from build123d import *

# Parameters (mm, degrees)
SKETCH1_W               = 30
SKETCH1_H               = 30
MAIN_BODY_DEPTH         = 11
SKETCH2_W               = 17.84
SKETCH2_H               = 2.8
WIRE_HOLE_DEPTH         = 6
BOARD_CAVITY_DEPTH      = 3
BOARD_CAVITY_DEPTH_BACK = 17.2
SKETCH3_W               = 20.5
SKETCH3_H               = 3.6
SKETCH4_W               = 10
SKETCH4_H               = 10
LIGHT_BOX_DEPTH         = 2
SKETCH5_R               = 1.5
CUT_EXTRUDE4_DEPTH      = 20
SKETCH7_W               = 20.5
SKETCH7_H               = 3.6
CUT_EXTRUDE5_DEPTH      = 1
BOSS_EXTRUDE1_DEPTH     = 30
BOSS_EXTRUDE2_START     = 0.6
SKETCH11_W              = 10
SKETCH11_H              = 10
SKETCH11_R              = 1.5
BOSS_EXTRUDE2_DEPTH     = 0.6
SKETCH12_W              = 44.814636294
SKETCH12_H              = 7.577756332
CUT_EXTRUDE6_DEPTH      = 40


with BuildPart() as part:
    # Sketch1 → Main Body (new body)
    with BuildSketch(Plane(origin=(0, 0, 0), x_dir=(1, 0, 0), z_dir=(0, 1, 0))):
        Rectangle(SKETCH1_W, SKETCH1_H)
    extrude(amount=MAIN_BODY_DEPTH)

    # Sketch2 → Wire Hole (cut)
    with BuildSketch(Plane.XZ):
        with Locations((0, 8.6)):
            Rectangle(SKETCH2_W, SKETCH2_H)
    extrude(amount=-WIRE_HOLE_DEPTH, mode=Mode.SUBTRACT)

    # Sketch3 → Board Cavity (cut, two sides: drawn at the far end of the back side and taken through both)
    with BuildSketch(Plane.XY.offset(7.2).offset(-BOARD_CAVITY_DEPTH_BACK)):
        with Locations((0, 4.2)):
            Rectangle(SKETCH3_W, SKETCH3_H)
    extrude(amount=BOARD_CAVITY_DEPTH + BOARD_CAVITY_DEPTH_BACK, mode=Mode.SUBTRACT)

    # Sketch4 → Light Box (cut)
    with BuildSketch(Plane.XZ.offset(-6)):
        with Locations((0, 0.05)):
            Rectangle(SKETCH4_W, SKETCH4_H)
    extrude(amount=-LIGHT_BOX_DEPTH, mode=Mode.SUBTRACT)

    # Sketch5 → Cut-Extrude4 (cut)
    with BuildSketch(Plane.XZ.offset(-8)):
        with Locations(Location((0, 0, 0), (0, 0, 270))):
            Circle(SKETCH5_R)
    extrude(amount=-CUT_EXTRUDE4_DEPTH, mode=Mode.SUBTRACT)

    # Sketch7 → Cut-Extrude5 (cut)
    with BuildSketch(Plane.XY.offset(-10)):
        with Locations((0, 4.2)):
            Rectangle(SKETCH7_W, SKETCH7_H)
    extrude(amount=-CUT_EXTRUDE5_DEPTH, mode=Mode.SUBTRACT)

    # Sketch8 → Boss-Extrude1 (add)
    with BuildSketch(Plane(origin=(0, 0, -15), x_dir=(-1, 0, 0), z_dir=(0, 0, -1))):
        Polygon((-15, 5.5), (-15, 3.8), (-17.2, 3.8), (-17.2, 2.5), (-19.75, 2.5), (-19.75, 8.5), (-17.2, 8.5), (-17.2, 7.2), (-15, 7.2), align=None)
    boss_extrude1 = extrude(amount=-BOSS_EXTRUDE1_DEPTH)

    # Mirror1: Boss-Extrude1 across plane
    add(boss_extrude1.mirror(Plane(origin=(0, 0, 0), x_dir=(0, 0, 1), z_dir=(1, 0, 0))))

    # Sketch9 → Cut-Revolve6 (revolve, cut)
    with BuildSketch(Plane.XY, mode=Mode.PRIVATE) as cut_revolve6_sk:
        with BuildLine():
            Line((0, 67.971820098), (0, 8))
            Line((0, 8), (-1.3, 8))
            ThreePointArc((-1.3, 8), (-29.992954197, 38.621972793), (0, 67.971820098))
        make_face()
    revolve(cut_revolve6_sk.sketch.rotate(Axis((0, 0, 0), (0, -1, 0)), 90), axis=Axis((0, 0, 0), (0, -1, 0)), mode=Mode.SUBTRACT)

    # Sketch11 → Boss-Extrude2 (add)
    with BuildSketch(Plane.XZ.offset(-8).offset(BOSS_EXTRUDE2_START)):
        with Locations((0, 0.05)):
            Rectangle(SKETCH11_W, SKETCH11_H)
        with Locations(Location((0, 0, 0), (0, 0, 270))):
            Circle(SKETCH11_R, mode=Mode.SUBTRACT)
    extrude(amount=-BOSS_EXTRUDE2_DEPTH)

    # Sketch12 → Cut-Extrude6 (cut)
    with BuildSketch(Plane(origin=(0, 0, -15), x_dir=(-1, 0, 0), z_dir=(0, 0, -1))):
        with Locations((-2.128069321, 9.788878166)):
            Rectangle(SKETCH12_W, SKETCH12_H)
    extrude(amount=-CUT_EXTRUDE6_DEPTH, mode=Mode.SUBTRACT)


solid = part.part
Could you check a few things on this model? Use its own coordinates, in mm. A direction names the side the tool comes from. Round coordinates to 2 decimals unless told otherwise and drop trailing zeros. Write each loop counter-clockwise with the first axis right and the second up, starting at its lowest first coordinate (ties: lowest second). Pieces come first, ordered by that corner, then holes. Notation, with made-up numbers: (15, -1) - (29, -1) arc R28 ccw to (29, 19) - close; hole circle Ø8 at (-24.5, 39). An arc over 180 degrees is marked (long way). Use a Markdown table: item, result.
Q1. Please list where these lines run through material, in increasing order: L1, parallel to X at y = 5.15, z = 9.25; L2, parallel to Z at x = 6, y = 3.9; L3, parallel to X at y = 3.5, z = -11.75.
Output values:
| item | result |
|---|---|
| L1 | -19.75 to -10.25, 10.25 to 19.75 |
| L2 | -15 to -11, 10.2 to 15 |
| L3 | -19.75 to -17.2, -15 to 15, 17.2 to 19.75 |
Q2. I want a section at A-A (y = 2.9). List the corners of the cut face in (x, z) for me, plus the area to 3 significant figures.
Output values:
| item | result |
|---|---|
| outline | (-19.75, -15) - (-17.2, -15) - (-17.2, 15) - (-19.75, 15) - close; (-15, -15) - (15, -15) - (15, 15) - (-15, 15) - close; (17.2, -15) - (19.75, -15) - (19.75, 15) - (17.2, 15) - close; hole (-10.25, -11) - (10.25, -11) - (10.25, 10.2) - (-10.25, 10.2) - close |
| area | 618 mm2 |
Q3. I want a section at B-B (x = -3). List the corners of the cut face in (y, z) for me, plus the area to 3 significant figures.
Output values:
| item | result |
|---|---|
| outline | (0, -15) - (6, -15) - (6, -11) - (2.4, -11) - (2.4, 7.2) - (0, 7.2) - close; (0, 10) - (2.4, 10) - (2.4, 10.2) - (6, 10.2) - (6, 15) - (0, 15) - close |
| area | 97.0 mm2 |
Q4. Thinking about a two-plate mould opening in X: for faces 6 (the flat face through (0, 3, -15)), 7 (the flat face through (-19.75, 4, 0)), 8 (the flat face through (-15, 2, 0)), 9 (the flat face through (19.75, 4, 0)), which applies, released by +X, released by -X, zero draft, split by the parting line, or undercut?
Output values:
| item | result |
|---|---|
| face 6 | zero draft |
| face 7 | released by -X |
| face 8 | undercut |
| face 9 | released by +X |
Q5. I want a section at C-C (z = 12.75). List the corners of the cut face in (x, y) for me, plus the area to 3 significant figures.
Output values:
| item | result |
|---|---|
| outline | (-19.75, 2.5) - (-17.2, 2.5) - (-17.2, 3.8) - (-15, 3.8) - (-15, 0) - (15, 0) - (15, 3.8) - (17.2, 3.8) - (17.2, 2.5) - (19.75, 2.5) - (19.75, 6) - (-19.75, 6) - close |
| area | 208 mm2 |
Q6. For pin 1 (16.5 mm diameter, centred on x = -1.5, z = -1.5, fed in from +Y); pin 2 (1.1 mm diameter, centred on x = 16.5, z = -0.5, fed in from -Y); pin 3 (0.7 mm diameter, centred on y = 1.5, z = 8.5, fed in from -X), each with a flat end and sliding along its axis, tell me the tip position at first contact or that it passes through.
Output values:
| item | result |
|---|---|
| pin 1 | y = 2.4 |
| pin 2 | y = 3.8 |
| pin 3 | x = -15 |
Q7. For faces 1 (the flat face through (16, 3.8, 0)), 2 (the flat face through (0, 2.4, -1)), 3 (the flat face through (-18, 2.5, 0)), 4 (the flat face through (0, 1, 7.2)), 5 (the flat face through (0, 0, 0)), which set-ups out of +Z, -Z, +X, -X, +Y, -Y let a thin tool reach every point of the face, with its end or its side?
Output values:
| item | result |
|---|---|
| face 1 | +Z, -Z, -Y |
| face 2 | +Y |
| face 3 | +Z, -Z, -X, -Y |
| face 4 | +Y, -Y |
| face 5 | +Z, -Z, +X, -X, -Y |
Q8. I want a section at D-D (y = 4.65). List the corners of the cut face in (x, z) for me.
Output values:
| item | result |
|---|---|
| outline | (-19.75, -15) - (19.75, -15) - (19.75, 15) - (-19.75, 15) - close; hole (-10.25, -11) - (10.25, -11) - (10.25, 10.2) - (-10.25, 10.2) - close |
